Verification items for this drawing (mm, ordinates from the low corner). Round coordinates to 2 decimals unless told otherwise and drop trailing zeros. Order: outer loops, then holes, each group sorted by start corner. A loop starts at its lowest first (then second) coordinate and runs counter-clockwise, first axis right, second up. Notation, with made-up numbers: (-39.75, -24) - (-35.75, -24) arc R9 ccw to (-35.75, -7) - close; hole circle Ø1 at (45, 82.5). An arc over 180 degrees is marked (long way). Answer as CSV lines item,"result". Start each with the question number.
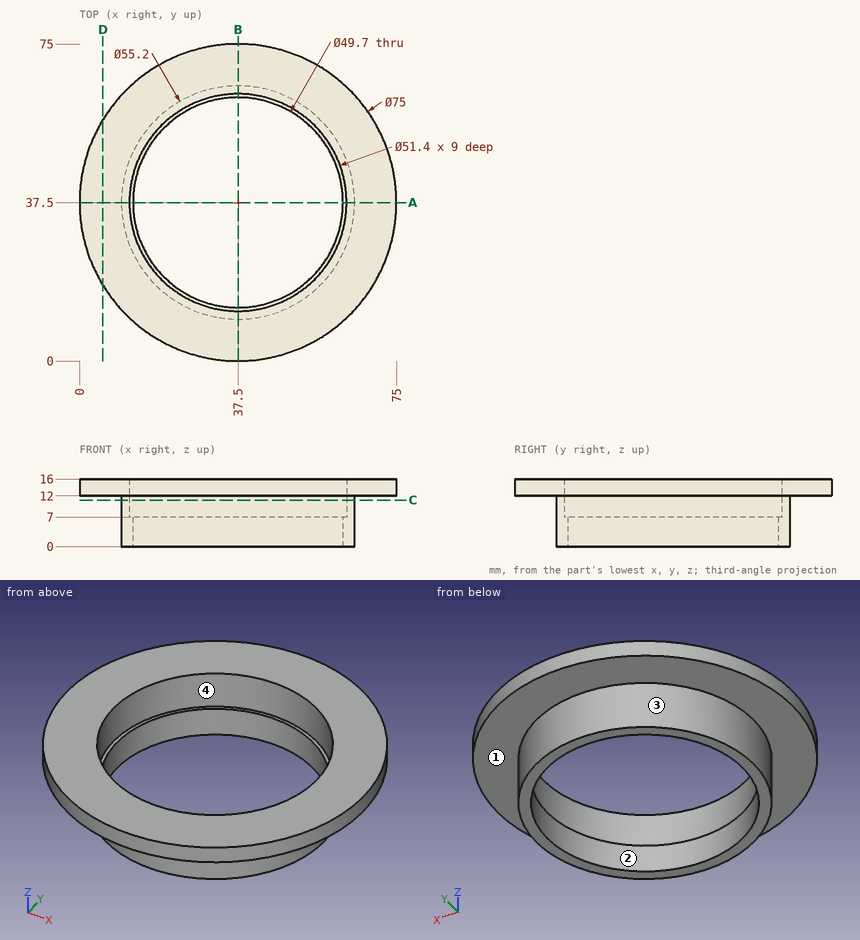
1. Thickness scan on probe 1 along Y at (x, z) = (37, 4.25); probe 2 along Y at (x, z) = (37.5, 12.75); probe 3 along Z at (x, y) = (69, 43). Record the ranges inside material, lowest first.
2. Section check A-A on y = 37.5. Record the boundary of the cut face in (x, z), plus the area to 3 significant figures.
3. Go/stop test with flat-tipped pins: pin 1 Ø2 at (x, z) = (66, 14) entering from -Y; pin 2 Ø8 at (x, z) = (14.5, 3) entering from +Y; pin 3 Ø3 at (x, z) = (31, 5) entering from +Y. Record where each tip stops, or that it passes through.
4. Section check D-D on x = 5.5. Record the boundary of the cut face in (y, z), plus the area to 3 significant figures.
5. Section check C-C on z = 11. Record the boundary of the cut face in (x, y), plus the area to 3 significant figures.
6. Draft check along X on the marked faces 1, 2, 3 and 4. Enter one of: released by +X, released by -X, zero draft, split by the parting line, or undercut.
Numbers:
1,probe 1,"y = 9.9 to 12.66, 62.34 to 65.1"
1,probe 2,"y = 0 to 11.8, 63.2 to 75"
1,probe 3,"z = 12 to 16"
2,outline,"(0, 12) - (9.9, 12) - (9.9, 0) - (12.65, 0) - (12.65, 7) - (11.8, 7) - (11.8, 16) - (0, 16) - close; (62.35, 0) - (65.1, 0) - (65.1, 12) - (75, 12) - (75, 16) - (63.2, 16) - (63.2, 7) - (62.35, 7) - close"
2,area,"152 mm2"
3,pin 1,"stops at y = 12"
3,pin 2,"stops at y = 57.52"
3,pin 3,"stops at y = 64.64"
4,outline,"(17.95, 12) - (57.05, 12) - (57.05, 16) - (17.95, 16) - close"
4,area,"156 mm2"
5,outline,"circle Ø55.2 at (37.5, 37.5); hole circle Ø51.4 at (37.5, 37.5)"
5,area,"318 mm2"
6,face 1,"zero draft"
6,face 2,"undercut"
6,face 3,"split by the parting line"
6,face 4,"undercut"
